Design review of the part built by this model. Coordinates are the model's own, in mm. A direction names the side the tool comes from. Round coordinates to 2 decimals unless told otherwise and drop trailing zeros. Loops run counter-clockwise (first coordinate to the right, second up) from the corner with the lowest first, then second, coordinate; pieces in that order, holes last. Notation, with made-up numbers: (-36.75, -40) -> (-28.75, -40) arc R19 ccw to (-28.75, -13) -> close; hole circle Ø3 at (-37, 42.5). An arc over 180 degrees is marked (long way). Use a Markdown table: item, result. Add a question column.
Autodesk Inventor part; units mm, degrees
ref_plane "YZ Plane" through (0, 0, 0) normal (1, 0, 0) x (0, 1, 0)
ref_plane "XZ Plane" through (0, 0, 0) normal (0, 1, 0) x (-1, 0, 0)
ref_plane "XY Plane" through (0, 0, 0) normal (0, 0, 1) x (1, 0, 0)
sketch "Sketch1" plane through (0, 0, 0) normal (0, 1, 0) x (-1, 0, 0)
  line L0 (40, 57.5) -> (-40, 57.5)
  line L1 (-40, 57.5) -> (-40, -57.5)
  line L2 (-40, -57.5) -> (40, -57.5)
  line L3 (40, -57.5) -> (40, 57.5)
  point P0 (0, 0)
  point P1 (40, 0)
  point P2 (0, 57.5)
  dimension "d0" = 115
  dimension "d1" = 80
extrude "Extrusion1" add sketch "Sketch1" along normal blind 20
sketch "Sketch12" plane through (0, 0, 0) normal (0, -1, 0) x (1, 0, 0)
  line L0 (-40, 57.5) -> (-20, 57.5)
  line L1 (-20, 57.5) -> (-20, -57.5)
  line L2 (-20, -57.5) -> (-40, -57.5)
  line L3 (-40, -57.5) -> (-40, 57.5)
  line L4 (-40, -57.5) -> (-40, 57.5)
  line L5 (0, 100.8809) -> (0, -116.5773) construction
  line L6 (40, 57.5) -> (20, 57.5)
  line L7 (20, 57.5) -> (20, -57.5)
  line L8 (20, -57.5) -> (40, -57.5)
  line L9 (40, -57.5) -> (40, 57.5)
  point P0 (0, 0)
  point P1 (-40, 0)
  point P2 (0, 0)
  point P3 (-20, 0)
  dimension "d56" = 20
  dimension "d57" = 115
extrude "Extrusion11" add sketch "Sketch12" along normal blind 37.5
sketch "Sketch13" plane through (-40, 0, 57.5) normal (-1, 0, 0) x (0, 0, 1)
  line L0 (0, 0) -> (-115, 0)
  point P0 (-57.5, 0)
  point P1 (-22.5, -15)
  point P2 (-92.5, -15)
  point P3 (-57.5, -15)
  point P4 (-57.5, 0)
  dimension "d129" = 35
  dimension "d130" = 35
  dimension "d131" = 15
hole "Hole2" at (-40, -15, 35) at (-40, -15, -35) direction (1, 0, 0) diameter 20 end through all
hole "Hole3" at (-40, -15, 0) direction (1, 0, 0) diameter 15 end through all
sketch "Sketch19" plane through (0, 20, 0) normal (0, 1, 0) x (1, 0, 0)
  point P0 (0, 0)
  point P1 (25, 0)
  point P2 (-25, 0)
  dimension "d111" = 25
  dimension "d112" = 25
hole "Hole6" at (25, 20, 0) at (-25, 20, 0) direction (0, -1, 0) diameter 15 depth 15
fillet "Fillet19" radius 20 4 edges at (-30, -37.5, -57.5) (30, -37.5, -57.5) (30, -37.5, 57.5) (-30, -37.5, 57.5)
sketch "Sketch20" plane through (0, 20, 0) normal (0, 1, 0) x (1, 0, 0)
  line L0 (-40, -57.5) -> (40, -57.5)
  line L1 (40, -57.5) -> (40, -47.5)
  line L2 (40, -47.5) -> (-40, -47.5)
  line L3 (-40, -47.5) -> (-40, -57.5)
  line L4 (-40, 57.5) -> (-40, -57.5)
  line L5 (40, -57.5) -> (40, 57.5)
  line L6 (-40, -57.5) -> (40, -57.5)
  point P0 (0, 0)
  dimension "d122" = 10
extrude "Extrusion15" add sketch "Sketch20" along normal blind 50
sketch "Sketch21" plane through (-40, 20, 57.5) normal (0, 0, 1) x (1, 0, 0)
  circle A0 centre (40, 25) radius 7.5
  line L0 (20, -20) -> (60, -20)
  line L1 (0, 50) -> (80, 50)
  circle A1 centre (40, 25) radius 11
  point P0 (40, -20)
  point P1 (40, -20)
  point P2 (0, -20)
  point P3 (80, -20)
  point P4 (24.5, 40.5)
  point P5 (24.5, 9.5)
  point P6 (55.5, 9.5)
  point P7 (55.5, 40.5)
  dimension "d128" = 15
  dimension "d132" = 25
  dimension "d134" = 15.5
  dimension "d135" = 15.5
  dimension "d138" = 360
  dimension "d147" = 22
extrude "Extrusion16" cut sketch "Sketch21" against normal blind 50 contours A0
fillet "Fillet20" radius 10 1 edges at (0, 20, 47.5)
hole "Hole7" at (-15.5, 60.5, 57.5) at (-15.5, 29.5, 57.5) at (15.5, 29.5, 57.5) at (15.5, 60.5, 57.5) direction (0, 0, -1) diameter 5 depth 15
extrude "Extrusion17" cut sketch "Sketch21" against normal blind 2
properties part number "Y_Slider_Part"
1. Consider section D-D on y = 60.5. State the section outline as (x, z) points, plus the area to 3 significant figures.
2. Consider section A-A on y = 45. State the section outline as (x, z) points, plus the area to 3 significant figures.
3. Insertion check: P1, Ø1.5, axis at x = -4, z = -44.5, coming from the -Y side; P2, Ø2, axis at x = -7.5, y = 40.5, coming from the -Z side; P3, Ø17.5, axis at x = 0, y = 45, coming from the +Z side; P4, Ø9, axis at y = -15, z = 0, coming from the +X side. Each pin has a flat end and moves straight along its axis. Give the tip position at first contact, or say it passes through.
4. Consider section B-B on z = 0. State the section outline as (x, y) points.
5. Consider section C-C on x = 0. State the section outline as (y, z) points.
6. For faces 5 (the face through (1, 20, -9)), 6 (the face through (17.564, 12.395, -0.976)), 7 (the face through (20, -23, 1)), list the 3-axis set-ups (+Z, -Z, +X, -X, +Y, -Y) from which the entire face can be reached by the end or side of a thin tool; tool diameter is ignored.
7. Mouldability with a two-part tool opening along Y and no side actions: class faces 1 (the face through (0, 0, 1)), 2 (the face through (-14, 31.5, 52.2)), 3 (the face through (16.46, 58.19, 52.43)), 4 (the face through (-1, 26, 57.5)) as +Y half, -Y half, draft (parallel to the pull), parting line (faces both ways), or undercut.
8. To check wall thickness, follow probe 1 along Z at (x, y) = (-33, -15); probe 2 along X at (y, z) = (29.5, 50); probe 3 along Y at (x, z) = (0, 50). State the ranges of each line that lie inside material, in increasing order. Write a range as from..to.
Verdict:
| question | item | result |
|---|---|---|
| 1 | outline | (-40, 47.5) -> (-18, 47.5) -> (-18, 57.5) -> (-40, 57.5) -> close; (-13, 47.5) -> (13, 47.5) -> (13, 57.5) -> (-13, 57.5) -> close; (18, 47.5) -> (40, 47.5) -> (40, 57.5) -> (18, 57.5) -> close |
| 1 | area | 700 mm² |
| 2 | outline | (-40, 47.5) -> (-7.5, 47.5) -> (-7.5, 55.5) -> (-11, 55.5) -> (-11, 57.5) -> (-40, 57.5) -> close; (7.5, 47.5) -> (40, 47.5) -> (40, 57.5) -> (11, 57.5) -> (11, 55.5) -> (7.5, 55.5) -> close |
| 2 | area | 636 mm² |
| 3 | P1 | stops at y = 0 |
| 3 | P2 | stops at z = 47.5 |
| 3 | P3 | stops at z = 55.5 |
| 3 | P4 | passes through |
| 4 | outline | (-40, -37.5) -> (-20, -37.5) -> (-20, -22.5) -> (-40, -22.5) -> close; (-40, -7.5) -> (-20, -7.5) -> (-20, 0) -> (20, 0) -> (20, -7.5) -> (40, -7.5) -> (40, 20) -> (32.5, 20) -> (32.5, 5) -> (17.5, 5) -> (17.5, 20) -> (-17.5, 20) -> (-17.5, 5) -> (-32.5, 5) -> (-32.5, 20) -> (-40, 20) -> close; (20, -37.5) -> (40, -37.5) -> (40, -22.5) -> (20, -22.5) -> close |
| 5 | outline | (0, -57.5) -> (20, -57.5) -> (20, 37.5) arc R10 cw to (30, 47.5) -> (37.5, 47.5) -> (37.5, 55.5) -> (34, 55.5) -> (34, 57.5) -> (0, 57.5) -> close; (52.5, 47.5) -> (70, 47.5) -> (70, 57.5) -> (56, 57.5) -> (56, 55.5) -> (52.5, 55.5) -> close |
| 6 | face 5 | -Z, +X, -X, +Y |
| 6 | face 6 | +Y |
| 6 | face 7 | +Z, -Z, -Y |
| 7 | face 1 | -Y half |
| 7 | face 2 | undercut |
| 7 | face 3 | undercut |
| 7 | face 4 | draft |
| 8 | probe 1 | z = -57.5..-45, -25..-7.5, 7.5..25, 45..57.5 |
| 8 | probe 2 | x = -40..-18, -13..13, 18..40 |
| 8 | probe 3 | y = 0..37.5, 52.5..70 |
